Input: part model. Units: mm. Frame: model coordinates. Face numbers are marked on the shaded views. A direction names the side the tool comes from. Give positions to 0.01 mm unless a question says otherwise; leave off trailing zeros. Loops run counter-clockwise (first coordinate to the right, second up) from the corner with the lowest first, then second, coordinate; pieces in that order, holes last. Notation, with made-up numbers: (80.5, 47) -> (114.5, 47) arc R13 ccw to (114.5, 58) -> close; hole circle Ø7 at (30.5, -14). An arc over 180 degrees is marked (long way). Answer in a Markdown table with one row per item. Add a question column.
```python
from build123d import *

# Parameters (mm, degrees)
SKETCH_1_W          = 62
SKETCH_1_H          = 35
EXTRUDE_1_DEPTH     = 1.5
SKETCH_2_W          = 62
SKETCH_2_H          = 35
EXTRUDE_2_DEPTH     = 30.629158
SKETCH_3_W          = 59
SKETCH_3_H          = 32
CUT_EXTRUDE_1_DEPTH = 41
SKETCH_4_W          = 62
SKETCH_4_H          = 35
SKETCH_4_W_2        = 59
SKETCH_4_H_2        = 32
EXTRUDE_3_DEPTH     = 1
SKETCH_5_W          = 62
SKETCH_5_H          = 35
EXTRUDE_4_DEPTH     = 1.5
SKETCH_8_R          = 5
CUT_EXTRUDE_3_DEPTH = 1.5
CUT_EXTRUDE_4_REACH = 36.629
SKETCH_10_W         = 14
SKETCH_10_H         = 14


with BuildPart() as part:
    # 草图1 → 凸台-拉伸1 (new body)
    with BuildSketch(Plane(origin=(0, 0, 0), x_dir=(1, 0, 0), z_dir=(0, 1, 0))):
        with Locations((2.996831225, 4.751847291)):
            Rectangle(SKETCH_1_W, SKETCH_1_H)
    extrude(amount=EXTRUDE_1_DEPTH)

    # 草图2 → 凸台-拉伸2 (add)
    with BuildSketch(Plane.XZ):
        with Locations((2.996831225, -4.751847291)):
            Rectangle(SKETCH_2_W, SKETCH_2_H)
    extrude(amount=EXTRUDE_2_DEPTH)

    # 草图3 → 切除-拉伸1 (cut)
    with BuildSketch(Plane.XZ.offset(30.629158461)):
        with Locations((2.996831225, -4.751847291)):
            Rectangle(SKETCH_3_W, SKETCH_3_H)
    extrude(amount=-CUT_EXTRUDE_1_DEPTH, mode=Mode.SUBTRACT)

    # 草图4 → 凸台-拉伸3 (add)
    with BuildSketch(Plane(origin=(0, 1.5, 0), x_dir=(1, 0, 0), z_dir=(0, 1, 0))):
        with Locations((2.996831225, 4.751847291)):
            Rectangle(SKETCH_4_W, SKETCH_4_H)
        with Locations((2.996831225, 4.751847291)):
            Rectangle(SKETCH_4_W_2, SKETCH_4_H_2, mode=Mode.SUBTRACT)
    extrude(amount=EXTRUDE_3_DEPTH)

    # 草图5 → 凸台-拉伸4 (add)
    with BuildSketch(Plane(origin=(0, 2.5, 0), x_dir=(1, 0, 0), z_dir=(0, 1, 0))):
        with Locations((2.996831225, 4.751847291)):
            Rectangle(SKETCH_5_W, SKETCH_5_H)
    extrude(amount=EXTRUDE_4_DEPTH)

    # 草图8 → 切除-拉伸3 (cut)
    with BuildSketch(Plane(origin=(33.996831225, 0, 0), x_dir=(0, 0, -1), z_dir=(1, 0, 0))):
        with Locations((4.751847291, -2.5)):
            Circle(SKETCH_8_R)
    extrude(amount=-CUT_EXTRUDE_3_DEPTH, mode=Mode.SUBTRACT)

    # 草图10 → 切除-拉伸4 (cut, up to next)
    with BuildSketch(Plane(origin=(0, 4, 0), x_dir=(1, 0, 0), z_dir=(0, 1, 0)), mode=Mode.PRIVATE) as cut_extrude_4_sk1:
        with Locations((2.996831225, 4.751847291)):
            Rectangle(SKETCH_10_W, SKETCH_10_H)
    cut_extrude_4_tool1 = extrude(cut_extrude_4_sk1.sketch, amount=-CUT_EXTRUDE_4_REACH, mode=Mode.PRIVATE) & part.part
    add(cut_extrude_4_tool1.solids().sort_by_distance((2.996831, 4, -4.751847))[0], mode=Mode.SUBTRACT)


solid = part.part
```
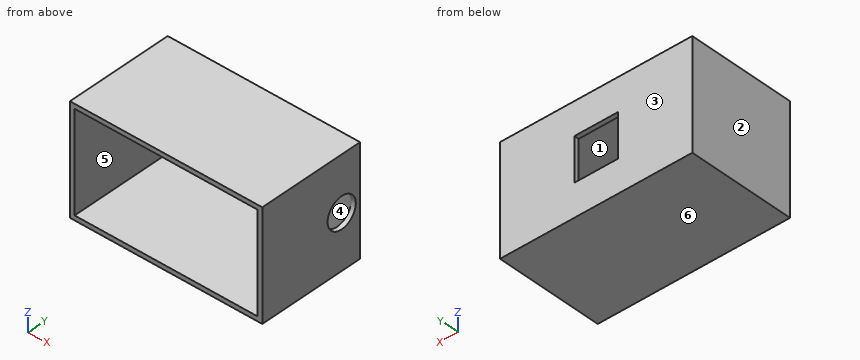
1) Section B-B on x = -2.5. Output: boundary loops of the cut face in (y, z).
2) Material intervals for line 1 along X through (y, z) = (-23, -3.5); line 2 along Z through (x, y) = (33.6, -2.5); line 3 along Z through (x, y) = (24.5, -2.5), sorted ascending.
3) Section A-A on y = -14. Output: boundary loops of the cut face in (x, z), and give its area (3 significant figures).
4) Section C-C on z = -1. Output: boundary loops of the cut face in (x, y).
5) Pin query (flat end, axial travel): pin 1 (6 mm diameter, centred on x = 4.5, z = -6.5, fed in from +Y); pin 2 (6 mm diameter, centred on x = 19, z = -5.5, fed in from -Y). Return the tip coordinate at first contact, or that it passes through.
6) Pull-direction query (X, two-part tool) for the marked faces 1, 2, 3 and 4; classes: +X half, -X half, draft (parallel to the pull), parting line (faces both ways), or undercut.
7) Reachability of the marked faces 5 and 6 from +Z, -Z, +X, -X, +Y, -Y: full face, straight path, thin tool, end or side. Return the list, or none.
8) Section D-D on z = 6.5. Output: boundary loops of the cut face in (x, y), and give its area (3 significant figures).
Working result:
| question | item | result |
|---|---|---|
| 1 | outline | (-30.63, -22.25) -> (4, -22.25) -> (4, -11.75) -> (2.5, -11.75) -> (2.5, -20.75) -> (-30.63, -20.75) -> close; (-30.63, 11.25) -> (2.5, 11.25) -> (2.5, 2.25) -> (4, 2.25) -> (4, 12.75) -> (-30.63, 12.75) -> close |
| 2 | line 1 | x = -28 to -26.5, 32.5 to 34 |
| 2 | line 2 | z = -22.25 to -9.75, 0.25 to 12.75 |
| 2 | line 3 | z = -22.25 to -20.75, 11.25 to 12.75 |
| 3 | outline | (-28, -22.25) -> (34, -22.25) -> (34, 12.75) -> (-28, 12.75) -> close; hole (-26.5, -20.75) -> (32.5, -20.75) -> (32.5, 11.25) -> (-26.5, 11.25) -> close |
| 3 | area | 282 mm2 |
| 4 | outline | (-28, -30.63) -> (-26.5, -30.63) -> (-26.5, 2.5) -> (-4, 2.5) -> (-4, 4) -> (-28, 4) -> close; (10, 2.5) -> (32.5, 2.5) -> (32.5, 0.81) -> (34, 0.81) -> (34, 4) -> (10, 4) -> close; (32.5, -30.63) -> (34, -30.63) -> (34, -5.81) -> (32.5, -5.81) -> close |
| 5 | pin 1 | passes through |
| 5 | pin 2 | stops at y = 2.5 |
| 6 | face 1 | undercut |
| 6 | face 2 | -X half |
| 6 | face 3 | draft |
| 6 | face 4 | undercut |
| 7 | face 5 | -Y |
| 7 | face 6 | -Z, +X, -X, +Y, -Y |
| 8 | outline | (-28, -30.63) -> (-26.5, -30.63) -> (-26.5, 2.5) -> (32.5, 2.5) -> (32.5, -30.63) -> (34, -30.63) -> (34, 4) -> (-28, 4) -> close |
| 8 | area | 192 mm2 |
